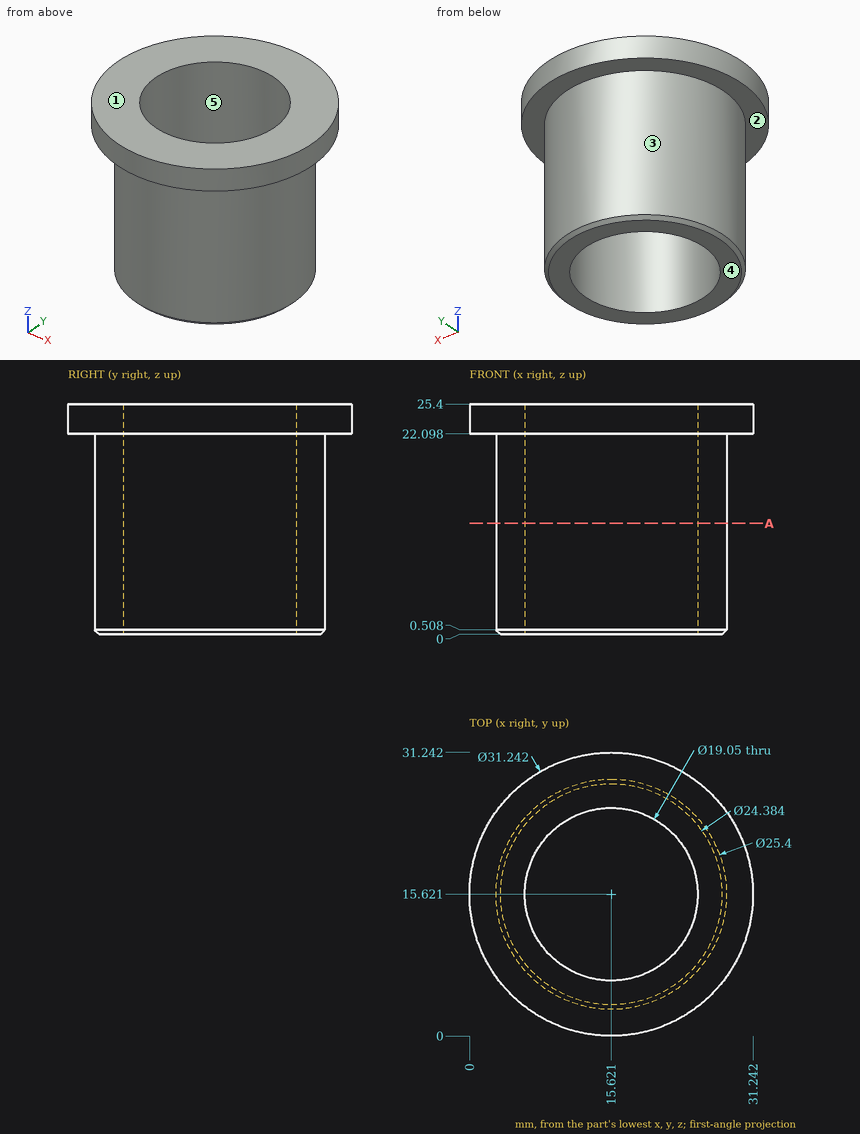
Input: dimensioned drawing with shaded views. Units: mm. Origin: part minimum x, y, z. A direction names the side the tool comes from. Round coordinates to 2 decimals unless told otherwise and drop trailing zeros. Loops run counter-clockwise (first coordinate to the right, second up) from the corner with the lowest first, then second, coordinate; pieces in that order, holes last. Notation, with made-up numbers: (87.5, -7) -> (93.5, -7) arc R22 cw to (93.5, 27) -> close; hole circle Ø1 at (16.25, -34). An arc over 180 degrees is marked (long way). Use one line per item in the form item = value. Start each with the question number.
1) Draft query along X for the marked faces 3, 4 and 5. Return one class per face: released by +X, released by -X, zero draft, split by the parting line, or undercut.
2) Section A-A on z = 12.25. Output: boundary loops of the cut face in (x, y) (3 decimals).
3) Line query: L1, parallel to X at y = 15.5, z = 3.5; L2, parallel to Z at x = 4, y = 10; L3, parallel to Y at x = 22.5, z = 9. Output: solid intervals per line, ascending.
4) First-contact query: P1, Ø4, axis at x = 21.5, z = 19.5, coming from the +Y side; P2, Ø4, axis at y = 22, z = 3, coming from the -X side; P3, Ø3, axis at y = 12.5, z = 22, coming from the -X side. Flat tips, straight axial feed; report the tip coordinate or a pass-through.
5) Access query for the marked faces 1 and 2. Directions: +Z, -Z, +X, -X, +Y, -Y. A direction counts if a zero-diameter tool reaches every point of the face in a straight line with its end or side. Return the directions, or none.
Response:
q1.face_3 = split by the parting line
q1.face_4 = zero draft
q1.face_5 = undercut
q2.outline = circle Ø25.4 at (15.621, 15.621); hole circle Ø19.05 at (15.621, 15.621)
q3.L1 = 2.92 to 6.1, 25.15 to 28.32
q3.L2 = 22.1 to 25.4
q3.L3 = 4.95 to 9.03, 22.21 to 26.3
q4.P1 = 27.71
q4.P2 = 3.7
q4.P3 = 0.08
q5.face_1 = +Z, +X, -X, +Y, -Y
q5.face_2 = -Z
